from build123d import *

# Parameters (mm, degrees)
F0_R          = 85
F1_DEPTH      = 20
F3_DEPTH      = 10
F3_DEPTH_BACK = 10
F5_DEPTH      = 30
F5_DEPTH_BACK = 30
F7_DEPTH      = 25


with BuildPart() as f1:
    # F0 (on Top) → F1 (new body)
    with BuildSketch(Plane.XY):
        Circle(F0_R)
    extrude(amount=-F1_DEPTH)

    # F2 (on Front) → F3 (join, two sides)
    with BuildSketch(Plane.XZ) as f3_sk:
        with BuildLine():
            ThreePointArc((-17.5, 12.5), (-30.303301, 17.803301), (-25, 5))
            ThreePointArc((-25, 5), (-19.696699, 7.196699), (-17.5, 12.5))
        make_face()
        with BuildLine():
            Line((-25, 0), (0, 0))
            ThreePointArc((0, 0), (-25, 25), (-50, 0))
            Line((-50, 0), (-25, 0))
        make_face()
        with BuildLine():
            ThreePointArc((-17.5, 12.5), (-19.696699, 7.196699), (-25, 5))
            ThreePointArc((-25, 5), (-30.303301, 17.803301), (-17.5, 12.5))
        make_face(mode=Mode.SUBTRACT)
    extrude(amount=F3_DEPTH)
    extrude(f3_sk.sketch, amount=-F3_DEPTH_BACK)

    # F4 (on Front) → F5 (join, two sides)
    with BuildSketch(Plane.XZ) as f5_sk:
        with BuildLine():
            ThreePointArc((69.1, 7.5), (62.100862, 10.399138), (65, 3.4))
            ThreePointArc((65, 3.4), (67.899138, 4.600862), (69.1, 7.5))
        make_face()
        with BuildLine():
            ThreePointArc((80, 0), (65, 15), (50, 0))
            Line((50, 0), (65, 0))
            Line((65, 0), (80, 0))
        make_face()
        with BuildLine():
            ThreePointArc((69.1, 7.5), (67.899138, 4.600862), (65, 3.4))
            ThreePointArc((65, 3.4), (62.100862, 10.399138), (69.1, 7.5))
        make_face(mode=Mode.SUBTRACT)
    extrude(amount=F5_DEPTH)
    extrude(f5_sk.sketch, amount=-F5_DEPTH_BACK)

    # F6 (on Top) → F7 (cut)
    with BuildSketch(Plane.XY):
        Polygon((0, 8.88), (0, 0), (0, -8.88), (150, -8.88), (150, 8.88), align=None)
    extrude(amount=F7_DEPTH, mode=Mode.SUBTRACT)


solid = f1.part
For this review, take the finished solid that the model builds, in its own axes (mm). A direction names the side the tool comes from. Round coordinates to 2 decimals unless told otherwise and drop trailing zeros. Loops run counter-clockwise (first coordinate to the right, second up) from the corner with the lowest first, then second, coordinate; pieces in that order, holes last. Notation, with made-up numbers: (0.25, 82) - (36.25, 82) arc R25 cw to (36.25, 105) - close; hole circle Ø4 at (28, -20). An arc over 180 degrees is marked (long way). Use one line per item in the form item = value.
Item 1: Clearance check with flat-ended pins moving along their axes: P1, Ø1.5, axis at x = -39.5, z = -4, coming from the +Y side; P2, Ø5, axis at y = -5.5, z = 14.5, coming from the -X side; P3, Ø3, axis at x = -61.5, z = -14.5, coming from the -Y side. State where each tip first meets the part, or that it passes through.
Answers:
P1 = 75.65
P2 = -46.93
P3 = -60.21
Item 2: For line 1 (Z direction, x = 65, y = -22.5); line 2 (Y direction, x = 68.5, z = 3.5); line 3 (Y direction, x = -34.5, z = 6.5), list the stretches that pass through material, from the lowest coordinate up.
Answers:
line_1 = -20 to 3.4, 11.6 to 15
line_2 = -30 to -8.88, 8.88 to 30
line_3 = -10 to 10
Item 3: Consider section A-A on y = 5.5. Write out the cut boundary in (x, z), then the cut area to 3 significant figures.
Answers:
outline = (-84.82, -20) - (84.82, -20) - (84.82, 0) - (0, 0) arc R25 ccw to (-50, 0) - (-84.82, 0) - close; hole circle Ø15 at (-25, 12.5)
area = 4,200 mm^2
Item 4: Consider section C-C on y = -23. Write out the cut boundary in (x, z).
Answers:
outline = (-81.83, -20) - (81.83, -20) - (81.83, 0) - (80, 0) arc R15 ccw to (50, 0) - (-81.83, 0) - close; hole circle Ø8.2 at (65, 7.5)
Item 5: Consider section B-B on z = -12.5. Write out the cut boundary in (x, y).
Answers:
outline = circle Ø170 at (0, 0)
Item 6: Tool access review of faces 1 (the flat face through (-25, 10, 4)), 2 (the flat face through (65, 30, 3)), 3 (the flat face through (65, 8.88, 2)), 4 (the flat face through (65, -30, 3)): name each direction out of +Z, -Z, +X, -X, +Y, -Y from which nothing blocks a thin tool from reaching the whole face with its end or side.
Answers:
face_1 = +Z, -X, +Y
face_2 = +Z, +X, -X, +Y
face_3 = +Z, +X
face_4 = +Z, +X, -X, -Y
Item 7: Consider section D-D on x = 42. Write out the cut boundary in (y, z), then the cut area to 3 significant figures.
Answers:
outline = (-73.9, -20) - (73.9, -20) - (73.9, 0) - (-73.9, 0) - close
area = 2,960 mm^2
